Here's how the part is built. I have some questions about the finished solid (model axes, mm). Face numbers are marked on the shaded views. A direction names the side the tool comes from. Give positions to 0.01 mm unless a question says otherwise; leave off trailing zeros. Loops run counter-clockwise (first coordinate to the right, second up) from the corner with the lowest first, then second, coordinate; pieces in that order, holes last. Notation, with made-up numbers: M -35,35 L -28,35 A26 ccw -28,63 Z; hole C 60.5,56.5 d9. An arc over 180 degrees is marked long. Answer as CSV lines item,"result". Start each with the question number.
Item 1: I want a section at B-B on z = -11.2. List the corners of the cut face in (x, y) for me.
Item 2: I want a section at C-C on z = -25. List the corners of the cut face in (x, y) for me, plus the area to 3 significant figures.
Item 3: I want a section at D-D on x = -18.35. List the corners of the cut face in (y, z) for me.
Item 4: Will these pins go through, and if not, where does the flat tip stop? P1, Ø6.5, axis at x = -11.5, z = -32, coming from the -Y side; P2, Ø2.5, axis at x = -18.35, z = -31.2, coming from the -Y side; P3, Ø12, axis at x = -10, z = -32, coming from the +Y side; P4, Ø4, axis at x = -10, z = -32, coming from the -Y side.
Item 5: If I drill on line 1 along X through (y, z) = (-0.8, -31.2); line 2 along Z through (x, y) = (3, 3); line 3 along Z through (x, y) = (-5, 2.5), over which ranges is the centre line in solid material (lowest first)? Write a range as from..to.
Item 6: I want a section at A-A on y = -2. Give the number of separate pieces and of enclosed holes in the cut face, plus the area to 3 significant figures.
Item 7: For the marked faces 1 and 2, which set-ups out of +Z, -Z, +X, -X, +Y, -Y let a thin tool reach every point of the face, with its end or its side?
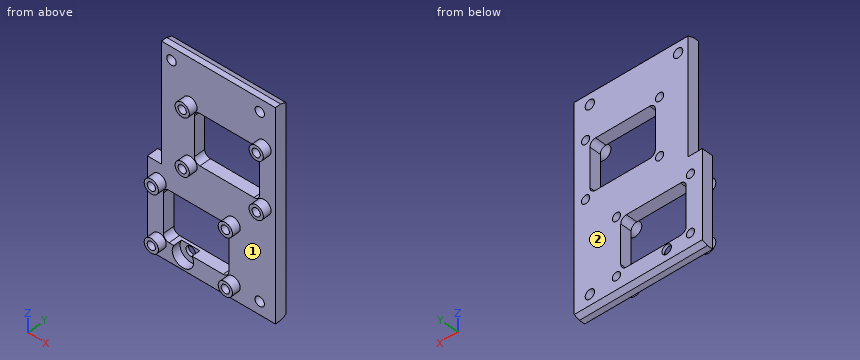
from build123d import *

# Parameters (mm, degrees)
SKETCH1_W             = 45
SKETCH1_H             = 74
SKETCH1_R             = 1.65
BOSS_EXTRUDE1_DEPTH   = 4
SKETCH3_R             = 3.75
CUT_EXTRUDE2_DEPTH    = 3
SKETCH4_W             = 5
SKETCH4_H             = 42
CUT_EXTRUDE3_DEPTH    = 5
SKETCH6_W             = 40
SKETCH6_H             = 0.5
SKETCH6_W_2           = 45
CUT_EXTRUDE4_DEPTH    = 5
CHAMFER1_SIZE         = 2
CHAMFER1_SIZE2        = 0.727940469
CHAMFER1_PART_2_SIZE  = 2
CHAMFER1_PART_2_SIZE2 = 0.727940469
SKETCH7_R             = 1.45
SKETCH7_W             = 23
SKETCH7_H             = 17.692307692
CUT_EXTRUDE5_DEPTH    = 5
FILLET1_R             = 2
SKETCH8_R             = 2.5
SKETCH8_R_2           = 1.45
BOSS_EXTRUDE2_DEPTH   = 3


with BuildPart() as part:
    # Sketch1 → Boss-Extrude1 (new body)
    with BuildSketch(Plane(origin=(0, 0, 0), x_dir=(1, 0, 0), z_dir=(0, 1, 0))):
        Rectangle(SKETCH1_W, SKETCH1_H)
        with Locations(Location((-10, 32, 0), (0, 0, 270))):  # turned: the seam where the file's is
            Circle(SKETCH1_R, mode=Mode.SUBTRACT)
        with Locations(Location((17, 32, 0), (0, 0, 270))):  # turned: the seam where the file's is
            Circle(SKETCH1_R, mode=Mode.SUBTRACT)
        with Locations(Location((-14, -32, 0), (0, 0, 270))):  # turned: the seam where the file's is
            Circle(SKETCH1_R, mode=Mode.SUBTRACT)
        with Locations(Location((17, -32, 0), (0, 0, 270))):  # turned: the seam where the file's is
            Circle(SKETCH1_R, mode=Mode.SUBTRACT)
    extrude(amount=BOSS_EXTRUDE1_DEPTH)

    # Sketch3 → Cut-Extrude2 (cut)
    with BuildSketch(Plane.XZ):
        with Locations(Location((-10, -32, 0), (0, 0, 270))):  # turned: the seam where the file's is
            Circle(SKETCH3_R)
    extrude(amount=-CUT_EXTRUDE2_DEPTH, mode=Mode.SUBTRACT)

    # Sketch4 → Cut-Extrude3 (cut, through all)
    with BuildSketch(Plane.XZ):
        with Locations((-20, 16)):
            Rectangle(SKETCH4_W, SKETCH4_H)
    extrude(amount=-CUT_EXTRUDE3_DEPTH, mode=Mode.SUBTRACT)

    # Sketch6 → Cut-Extrude4 (cut, through all)
    with BuildSketch(Plane.XZ):
        with Locations((2.5, 36.75)):
            Rectangle(SKETCH6_W, SKETCH6_H)
        with Locations((0, -36.75)):
            Rectangle(SKETCH6_W_2, SKETCH6_H)
    extrude(amount=-CUT_EXTRUDE4_DEPTH, mode=Mode.SUBTRACT)

    # Chamfer1
    chamfer1_edges = [part.edges().sort_by_distance(p)[0] for p in [
        (2.5, 4, 36.5),
    ]]
    chamfer1_side = [part.faces().sort_by_distance(p)[0] for p in [
        (2.5, 2, 36.5),
    ]]
    chamfer(chamfer1_edges, length=CHAMFER1_SIZE, length2=CHAMFER1_SIZE2, reference=chamfer1_side[0])

    # Chamfer1 part 2
    chamfer1_part_2_edges = [part.edges().sort_by_distance(p)[0] for p in [
        (0, 4, -36.5),
    ]]
    chamfer1_part_2_side = [part.faces().sort_by_distance(p)[0] for p in [
        (0, 2, -36.5),
    ]]
    chamfer(chamfer1_part_2_edges, length=CHAMFER1_PART_2_SIZE, length2=CHAMFER1_PART_2_SIZE2, reference=chamfer1_part_2_side[0])

    # Sketch7 → Cut-Extrude5 (cut, through all)
    with BuildSketch(Plane.XZ):
        with Locations(Location((-18.35, -31.2, 0), (0, 0, 270))):  # turned: the seam where the file's is
            Circle(SKETCH7_R)
        with Locations(Location((-18.35, -11.2, 0), (0, 0, 270))):  # turned: the seam where the file's is
            Circle(SKETCH7_R)
        with Locations(Location((7.65, -11.2, 0), (0, 0, 270))):  # turned: the seam where the file's is
            Circle(SKETCH7_R)
        with Locations(Location((7.65, -31.2, 0), (0, 0, 270))):  # turned: the seam where the file's is
            Circle(SKETCH7_R)
        with Locations(Location((18.5, 0.8, 0), (0, 0, 270))):  # turned: the seam where the file's is
            Circle(SKETCH7_R)
        with Locations(Location((-7.5, 0.8, 0), (0, 0, 270))):  # turned: the seam where the file's is
            Circle(SKETCH7_R)
        with Locations(Location((-7.5, 20.8, 0), (0, 0, 270))):  # turned: the seam where the file's is
            Circle(SKETCH7_R)
        with Locations(Location((18.5, 20.8, 0), (0, 0, 270))):  # turned: the seam where the file's is
            Circle(SKETCH7_R)
        with Locations((-5.35, -21.2)):
            Rectangle(SKETCH7_W, SKETCH7_H)
        with Locations((5.5, 10.8)):
            Rectangle(SKETCH7_W, SKETCH7_H)
    extrude(amount=-CUT_EXTRUDE5_DEPTH, mode=Mode.SUBTRACT)

    # Fillet1
    fillet1_edges = [part.edges().sort_by_distance(p)[0] for p in [
        (6.15, 2, -30.046153846),
        (-16.85, 2, -30.046153846),
        (-16.85, 2, -12.353846154),
        (6.15, 2, -12.353846154),
        (-6, 2, 1.953846154),
        (-6, 2, 19.646153846),
        (17, 2, 19.646153846),
        (17, 2, 1.953846154),
    ]]
    fillet(fillet1_edges, radius=FILLET1_R)

    # Sketch8 → Boss-Extrude2 (add)
    with BuildSketch(Plane.XZ):
        with Locations(Location((-18.35, -11.2, 0), (0, 0, 90))):  # turned: the seam where the file's is
            Circle(SKETCH8_R)
        with Locations(Location((-18.35, -11.2, 0), (0, 0, 270))):  # turned: the seam where the file's is
            Circle(SKETCH8_R_2, mode=Mode.SUBTRACT)
        with Locations(Location((-18.35, -31.2, 0), (0, 0, 90))):  # turned: the seam where the file's is
            Circle(SKETCH8_R)
        with Locations(Location((-18.35, -31.2, 0), (0, 0, 270))):  # turned: the seam where the file's is
            Circle(SKETCH8_R_2, mode=Mode.SUBTRACT)
        with Locations(Location((7.65, -11.2, 0), (0, 0, 90))):  # turned: the seam where the file's is
            Circle(SKETCH8_R)
        with Locations(Location((7.65, -11.2, 0), (0, 0, 270))):  # turned: the seam where the file's is
            Circle(SKETCH8_R_2, mode=Mode.SUBTRACT)
        with Locations(Location((7.65, -31.2, 0), (0, 0, 90))):  # turned: the seam where the file's is
            Circle(SKETCH8_R)
        with Locations(Location((7.65, -31.2, 0), (0, 0, 270))):  # turned: the seam where the file's is
            Circle(SKETCH8_R_2, mode=Mode.SUBTRACT)
        with Locations(Location((18.5, 0.8, 0), (0, 0, 90))):  # turned: the seam where the file's is
            Circle(SKETCH8_R)
        with Locations(Location((18.5, 0.8, 0), (0, 0, 270))):  # turned: the seam where the file's is
            Circle(SKETCH8_R_2, mode=Mode.SUBTRACT)
        with Locations(Location((-7.5, 0.8, 0), (0, 0, 90))):  # turned: the seam where the file's is
            Circle(SKETCH8_R)
        with Locations(Location((-7.5, 0.8, 0), (0, 0, 270))):  # turned: the seam where the file's is
            Circle(SKETCH8_R_2, mode=Mode.SUBTRACT)
        with Locations(Location((-7.5, 20.8, 0), (0, 0, 90))):  # turned: the seam where the file's is
            Circle(SKETCH8_R)
        with Locations(Location((-7.5, 20.8, 0), (0, 0, 270))):  # turned: the seam where the file's is
            Circle(SKETCH8_R_2, mode=Mode.SUBTRACT)
        with Locations(Location((18.5, 20.8, 0), (0, 0, 90))):  # turned: the seam where the file's is
            Circle(SKETCH8_R)
        with Locations(Location((18.5, 20.8, 0), (0, 0, 270))):  # turned: the seam where the file's is
            Circle(SKETCH8_R_2, mode=Mode.SUBTRACT)
    extrude(amount=BOSS_EXTRUDE2_DEPTH)


solid = part.part
Result:
1,outline,"M -22.5,0 L -20.85,0 L -20.85,-3 L -19.8,-3 L -19.8,4 L -22.5,4 Z; M -16.9,-3 L -15.85,-3 L -15.85,0 L 5.15,0 L 5.15,-3 L 6.2,-3 L 6.2,4 L -16.9,4 Z; M 9.1,-3 L 10.15,-3 L 10.15,0 L 22.5,0 L 22.5,4 L 9.1,4 Z"
2,outline,"M -22.5,0 L -16.85,0 L -16.85,4 L -22.5,4 Z; M 6.15,0 L 22.5,0 L 22.5,4 L 6.15,4 Z"
2,area,"88.0 mm^2"
3,outline,"M -3,-33.7 L 0,-33.7 L 0,-36.5 L 2,-36.5 L 4,-35.77 L 4,-32.65 L -3,-32.65 Z; M -3,-29.75 L 4,-29.75 L 4,-12.65 L -3,-12.65 L -3,-13.7 L 0,-13.7 L 0,-28.7 L -3,-28.7 Z; M -3,-9.75 L 4,-9.75 L 4,-5 L 0,-5 L 0,-8.7 L -3,-8.7 Z"
4,P1,"y = 0"
4,P2,"through"
4,P3,"y = 4"
4,P4,"y = 3"
5,line 1,"-20.85..-19.8, -16.9..-15.85, 5.15..6.2, 9.1..10.15"
5,line 2,"-36.14..-30.05, -12.35..1.95, 19.65..36.14"
5,line 3,"-36.32..-30.05, -12.35..2.22, 19.38..36.32"
6,separate pieces,"8"
6,enclosed holes,"8"
6,area,"104 mm^2"
7,face 1,"-Y"
7,face 2,"+Z, -Z, +X, -X, +Y"
